Here's how the part is built. I have some questions about the finished solid (model axes, mm). Face numbers are marked on the shaded views. Give positions to 0.01 mm unless a question says otherwise; leave off trailing zeros. Write each loop counter-clockwise with the first axis right and the second up, starting at its lowest first coordinate (ties: lowest second). Pieces come first, ordered by that corner, then holes. Notation, with made-up numbers: (-35.75, 46) - (-16.75, 46) arc R21 cw to (-16.75, 73) - close; hole circle Ø5 at (63, 21). An arc over 180 degrees is marked (long way). One line per item, written item: value. Start each with the question number.
1) Imagine slicing it at A-A on z = 2.25. Write out the boundary of the cut face in (x, y).
2) Please list where these lines run through material, in increasing order: L1, parallel to Y at x = 1.9, z = 16.5; L2, parallel to X at y = -0.4, z = 3.25; L3, parallel to Z at x = -0.2, y = 0.1. Write a range as [from, to].
3) We'd pull the mould along X, two halves only. Please class the marked faces 1 and 2: +X half, -X half, draft (parallel to the pull), parting line (faces both ways), or undercut.
4) Imagine slicing it at B-B on z = 20.5. Write out the boundary of the cut face in (x, y), plus the area to 3 significant figures.
5) I'm going to push flat-ended pins straight in: P1, Ø1.2, axis at x = -0.5, y = 0.5, coming from the -Z side; P2, Ø2, axis at x = -1.5, z = 8.5, coming from the -Y side. Where does each tip first touch, or does it pass through?
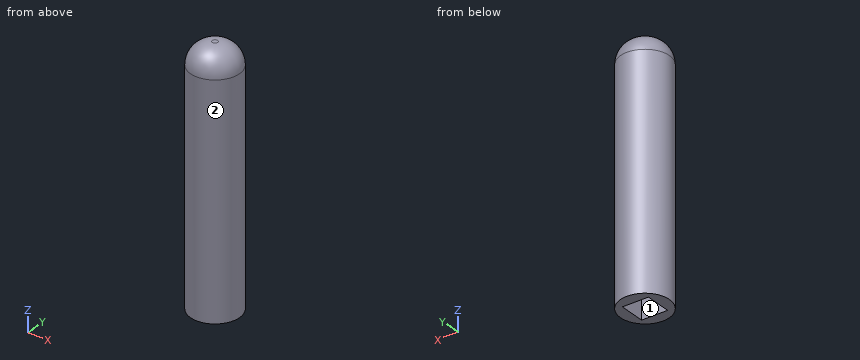
from build123d import *

# Parameters (mm, degrees)
SKETCH_1_R          = 2.25
EXTRUDE_2_DEPTH     = 23
SKETCH_7_W          = 2.4
SKETCH_7_H          = 2.4
CUT_EXTRUDE_3_DEPTH = 4.5
FILLET_2_R          = 2


with BuildPart() as part:
    # 草图1 → 凸台-拉伸2 (new body)
    with BuildSketch(Plane.XY):
        Circle(SKETCH_1_R)
    extrude(amount=EXTRUDE_2_DEPTH)

    # 草图7 → 切除-拉伸3 (cut)
    with BuildSketch(Plane.XY):
        Rectangle(SKETCH_7_W, SKETCH_7_H)
    extrude(amount=CUT_EXTRUDE_3_DEPTH, mode=Mode.SUBTRACT)

    # 圆角2
    fillet_2_edges = [part.edges().sort_by_distance(p)[0] for p in [
        (-2.25, 0, 23),
    ]]
    fillet(fillet_2_edges, radius=FILLET_2_R)


solid = part.part
Numbers:
1. outline: circle Ø4.5 at (0, 0); hole (-1.2, -1.2) - (1.2, -1.2) - (1.2, 1.2) - (-1.2, 1.2) - close
2. L1: [-1.21, 1.21]
2. L2: [-2.21, -1.2], [1.2, 2.21]
2. L3: [4.5, 23]
3. face 1: undercut
3. face 2: parting line
4. outline: circle Ø4.5 at (0, 0)
4. area: 15.9 mm^2
5. P1: z = 4.5
5. P2: y = -2.19
